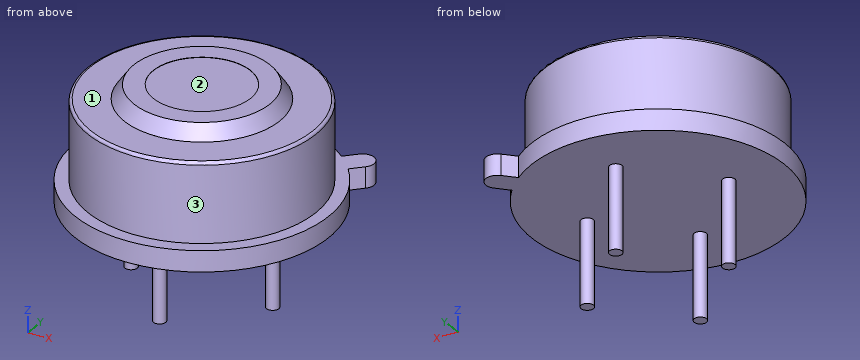
```python
from build123d import *

# Parameters (mm, degrees)
EXTRUDE_1_DEPTH     = 0.75
SKETCH_2_R          = 4.1
EXTRUDE_2_DEPTH     = 2.85
SKETCH_3_R          = 2.8
EXTRUDE_3_DEPTH     = 0.5
SKETCH_4_R          = 1.75
CUT_EXTRUDE_1_DEPTH = 0.01
FILLET_1_R          = 0.1
CHAMFER_1_SIZE2     = 0.350103769
CHAMFER_1_SIZE      = 0.5
SKETCH_5_R          = 0.225
EXTRUDE_4_DEPTH     = 3


with BuildPart() as part:
    # Эскиз1 → Бобышка-Вытянуть1 (new body)
    with BuildSketch(Plane.XY):
        with BuildLine():
            Line((2.91371601, 3.507685706), (3.309259736, 3.903229432))
            ThreePointArc((3.309259736, 3.903229432), (3.903229432, 3.903229432), (3.903229432, 3.309259736))
            Line((3.903229432, 3.309259736), (3.507685706, 2.91371601))
            ThreePointArc((3.507685706, 2.91371601), (-3.224406922, -3.224406922), (2.91371601, 3.507685706))
        make_face()
    extrude(amount=EXTRUDE_1_DEPTH)

    # Эскиз2 → Бобышка-Вытянуть2 (add)
    with BuildSketch(Plane.XY.offset(0.75)):
        Circle(SKETCH_2_R)
    extrude(amount=EXTRUDE_2_DEPTH)

    # Эскиз3 → Бобышка-Вытянуть3 (add)
    with BuildSketch(Plane.XY.offset(3.6)):
        Circle(SKETCH_3_R)
    extrude(amount=EXTRUDE_3_DEPTH)

    # Эскиз4 → Вырез-Вытянуть1 (cut)
    with BuildSketch(Plane.XY.offset(4.1)):
        Circle(SKETCH_4_R)
    extrude(amount=-CUT_EXTRUDE_1_DEPTH, mode=Mode.SUBTRACT)

    # Скругление1
    fillet_1_edges = [part.edges().sort_by_distance(p)[0] for p in [
        (-4.1, 0, 3.6),
    ]]
    fillet(fillet_1_edges, radius=FILLET_1_R)

    # Фаска1
    chamfer_1_edges = [part.edges().sort_by_distance(p)[0] for p in [
        (-2.8, 0, 4.1),
    ]]
    chamfer_1_side = [part.faces().sort_by_distance(p)[0] for p in [
        (-2.8, 0, 4.092997925),
    ]]
    chamfer(chamfer_1_edges, length=CHAMFER_1_SIZE - 0.0001, length2=CHAMFER_1_SIZE2 - 0.0001, reference=chamfer_1_side[0])  # a hair under: the kernel refuses the full size

    # Эскиз5 → Бобышка-Вытянуть4 (add)
    with BuildSketch(Plane(origin=(0, 0, 0), x_dir=(-1, 0, 0), z_dir=(0, 0, -1))):
        with Locations((-2.54, 0)):
            Circle(SKETCH_5_R)
        with Locations((0, -2.54)):
            Circle(SKETCH_5_R)
        with Locations((2.54, 0)):
            Circle(SKETCH_5_R)
        with Locations((0, 2.54)):
            Circle(SKETCH_5_R)
    extrude(amount=EXTRUDE_4_DEPTH)


solid = part.part
```
Geometry check sheet. Reference: the model listing, model coordinates, mm. Face numbers are marked on the shaded views. Round coordinates to 2 decimals unless told otherwise and drop trailing zeros. Loops run counter-clockwise (first coordinate to the right, second up) from the corner with the lowest first, then second, coordinate; pieces in that order, holes last. Notation, with made-up numbers: M -19.75,30 L 20.25,30 A26 cw 20.25,52 Z; hole C -3.75,0.25 d4. An arc over 180 degrees is marked long. Return JSON: item names as keys, results as strings. Group by question number.
(1) Section check B-B, the plane z = 2.75. Enter the section's corners in (x, y).
(2) Go/stop test with flat-tipped pins: pin 1 (2 mm diameter, centred on y = -3, z = 2, fed in from +X); pin 2 (3 mm diameter, centred on x = 0, y = 0, fed in from +Z); pin 3 (4 mm diameter, centred on x = -2.5, z = 0.5, fed in from -Y). Record where each tip stops, or that it passes through.
(3) Section check A-A, the plane z = -0.5. Enter the section's corners in (x, y) (3 decimals), and give its area (3 significant figures).
(4) Scan lines: line 1 along Z through (x, y) = (2.75, -3.5); line 2 along Z through (x, y) = (0.75, -1); line 3 along X through (y, z) = (-2.5, 1.5). Record each from-to range of solid material in increasing order. Write a range as [from, to].
(5) Mould release check, pull along Y, two halves, no side actions. Record for the marked faces 1, 2 and 3: pulls with the +Y half, pulls with the -Y half, needs draft (parallel to the pull), parting line crosses it, or undercut.
(6) Section check C-C, the plane y = 4.25. Enter the section's corners in (x, z).
Data:
{
 "1": {"outline": "C 0,0 d8.2"},
 "2": {"pin 1": "x = 3.58", "pin 2": "z = 4.09", "pin 3": "y = -4.53"},
 "3": {"outline": "C -2.54,0 d0.45; C 0,-2.54 d0.45; C 0,2.54 d0.45; C 2.54,0 d0.45", "area": "0.636 mm²"},
 "4": {"line 1": "[0, 0.75]", "line 2": "[0, 4.09]", "line 3": "[-3.25, 3.25]"},
 "5": {"face 1": "needs draft", "face 2": "undercut", "face 3": "parting line crosses it"},
 "6": {"outline": "M -1.65,0 L 1.65,0 L 1.65,0.75 L -1.65,0.75 Z"}
}
